CAD build for the part. Positions are in the model's coordinates, mm. Face numbers are marked on the shaded views. A direction names the side the tool comes from. Give positions to 0.01 mm unless a question says otherwise; leave off trailing zeros. Order: outer loops, then holes, each group sorted by start corner. A loop starts at its lowest first (then second) coordinate and runs counter-clockwise, first axis right, second up.
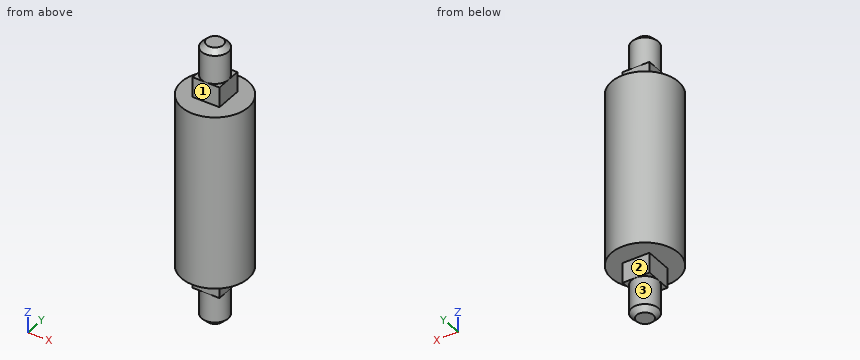
from build123d import *

# Parameters (mm, degrees)
SKIZZE1_R                       = 10
AUFSATZ_LINEAR_AUSTRAGEN1_DEPTH = 26
SKIZZE2_W                       = 8
SKIZZE2_H                       = 8
AUFSATZ_LINEAR_AUSTRAGEN2_DEPTH = 6
SKIZZE3_R                       = 4
AUFSATZ_LINEAR_AUSTRAGEN3_DEPTH = 10
FASE1_SIZE                      = 1.5


with BuildPart() as part:
    # Skizze1 → Aufsatz-Linear austragen1 (new body)
    with BuildSketch(Plane.XY):
        with Locations(Location((0, 0, 0), (0, 0, 180))):
            Circle(SKIZZE1_R)
    extrude(amount=AUFSATZ_LINEAR_AUSTRAGEN1_DEPTH)

    # Skizze2 → Aufsatz-Linear austragen2 (add)
    with BuildSketch(Plane.XY.offset(26)):
        Rectangle(SKIZZE2_W, SKIZZE2_H)
    extrude(amount=AUFSATZ_LINEAR_AUSTRAGEN2_DEPTH)

    # Skizze3 → Aufsatz-Linear austragen3 (add)
    with BuildSketch(Plane.XY.offset(32)):
        Circle(SKIZZE3_R)
    extrude(amount=AUFSATZ_LINEAR_AUSTRAGEN3_DEPTH)

    # Fase1
    fase1_edges = [part.edges().sort_by_distance(p)[0] for p in [
        (-4, 0, 42),
    ]]
    chamfer(fase1_edges, length=FASE1_SIZE)

    # Spiegeln1: part across plane


with BuildPart() as part_1:
    add(part.part)
    add(part.part.mirror(Plane.XY))


solid = part_1.part
1. Saw through at A-A on z = 24.5. Give the cut face in (x, y), plus the area to 3 significant figures.
2. 3-axis set-ups, long thin cutter, end or side, ignore diameter. For the marked faces 1, 2 and 3: which of +Z, -Z, +X, -X, +Y, -Y reach the whole face in a straight line?
3. Wall check: line 1 (Z direction, x = 6.25, y = 6); line 2 (Y direction, x = 3.75, z = -28.5); line 3 (Z direction, x = -3.5, y = 2). Give the ranges that are in metal, low to high.
4. Saw through at C-C on y = 6.75. Give the cut face in (x, z).
5. Pin check, flat tips, straight feed: P1, Ø1.2, axis at x = 3, y = 1, coming from the +Z side; P2, Ø3, axis at y = 4, z = 7, coming from the -X side; P3, Ø1.5, axis at x = -2, y = 7, coming from the +Z side. Stop position of each tip, or through.
6. Saw through at B-B on x = -6. Give the cut face in (y, z), plus the area to 3 significant figures.
Reported:
1. outline: circle Ø20 at (0, 0)
1. area: 314 mm2
2. face 1: +Z, +X, -X, -Y
2. face 2: -Z, +X, -X, +Y
2. face 3: -Z
3. line 1: z = -26 to 26
3. line 2: y = -4 to 4
3. line 3: z = -32 to 32
4. outline: (-7.38, -26) - (7.38, -26) - (7.38, 26) - (-7.38, 26) - close
5. P1: stops at z = 41.94
5. P2: stops at x = -9.68
5. P3: stops at z = 26
6. outline: (-8, -26) - (8, -26) - (8, 26) - (-8, 26) - close
6. area: 832 mm2
